Geometry check sheet. Reference: the model listing, model coordinates, mm. Face numbers are marked on the shaded views. A direction names the side the tool comes from. Coordinates: 2 decimals unless noted, no trailing zeros. Write each loop counter-clockwise with the first axis right and the second up, starting at its lowest first coordinate (ties: lowest second). Pieces come first, ordered by that corner, then holes. Notation, with made-up numbers: (35, 34.5) -> (94, 34.5) arc R8 ccw to (94, 38.5) -> close; hole circle Ø7 at (19.25, 16). An arc over 180 degrees is marked (long way). Use a Markdown table: item, result.
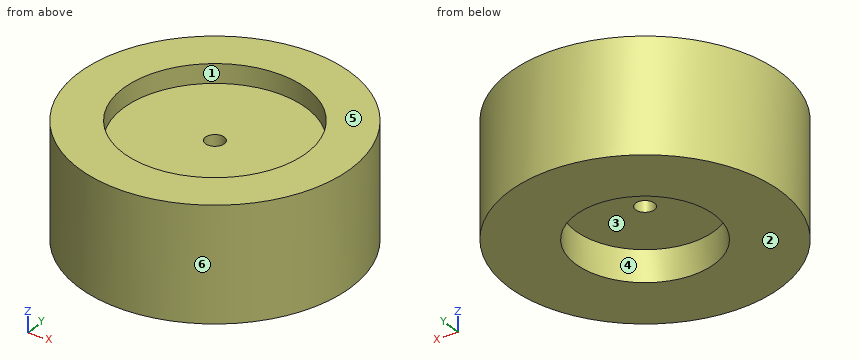
Autodesk Fusion 360 part; units mm, degrees
sketch "Esquisse1" plane through (0, 0, 0) normal (0, 0, 1) x (1, 0, 0)
  circle A0 centre (0, 0) radius 2.15
  dimension "d1" = 4.3
extrude "Extrusion1" add sketch "Esquisse1" along normal blind 1.8
sketch "Esquisse2" plane through (0, 0, 1.8) normal (0, 0, 1) x (-1, 0, 0)
  circle A0 centre (0, 0) radius 2.15
  circle A1 centre (0, 0) radius 1.45
  dimension "d4" = 2.9
extrude "Extrusion2" cut sketch "Esquisse2" against normal blind 0.3 contours A1
sketch "Esquisse3" plane through (0, 0, 0) normal (0, 0, -1) x (1, 0, 0)
  circle A0 centre (0, 0) radius 2.15
  circle A1 centre (0, 0) radius 1.1
  dimension "d7" = 2.2
extrude "Extrusion3" cut sketch "Esquisse3" against normal blind 0.5 contours A1
sketch "Esquisse4" plane through (0, 0, 1.5) normal (0, 0, 1) x (-1, 0, 0)
  circle A0 centre (0, 0) radius 1.45
  circle A1 centre (0, 0) radius 0.15
  dimension "d10" = 0.3
extrude "Extrusion4" cut sketch "Esquisse4" against normal blind 3.8 contours A1
scale "Echelle1" factor 10 about (1.45, 0, 1.8) bodies 1
Item 1: Section check D-D on x = -22. Record the boundary of the cut face in (y, z).
Answer block:
| item | result |
|---|---|
| outline | (-19.55, -16.2) -> (-6.4, -16.2) -> (-6.4, -11.2) -> (6.4, -11.2) -> (6.4, -16.2) -> (19.55, -16.2) -> (19.55, 1.8) -> (11.41, 1.8) -> (11.41, -1.2) -> (-11.41, -1.2) -> (-11.41, 1.8) -> (-19.55, 1.8) -> close |
Item 2: Mould release check, pull along X, two halves, no side actions. Record for the marked faces 4, 5 and 6: +X half, -X half, draft (parallel to the pull), parting line (faces both ways), or undercut.
Answer block:
| item | result |
|---|---|
| face 4 | undercut |
| face 5 | draft |
| face 6 | parting line |
Item 3: Section check A-A on y = 0. Record the boundary of the cut face in (x, z), then the cut area to 3 significant figures.
Answer block:
| item | result |
|---|---|
| outline | (-34.55, -16.2) -> (-24.05, -16.2) -> (-24.05, -11.2) -> (-14.55, -11.2) -> (-14.55, -1.2) -> (-27.55, -1.2) -> (-27.55, 1.8) -> (-34.55, 1.8) -> close; (-11.55, -11.2) -> (-2.05, -11.2) -> (-2.05, -16.2) -> (8.45, -16.2) -> (8.45, 1.8) -> (1.45, 1.8) -> (1.45, -1.2) -> (-11.55, -1.2) -> close |
| area | 547 mm^2 |
Item 4: Thickness scan on L1, parallel to Y at x = -13, z = -5.5; L2, parallel to Y at x = -13.05, z = 0.1; L3, parallel to Z at x = -24.5, y = -6.5. Record the ranges inside material, lowest first. Write a range as [from, to].
Answer block:
| item | result |
|---|---|
| L1 | y = [-21.5, -1.5], [1.5, 21.5] |
| L2 | y = [-21.5, -14.5], [14.5, 21.5] |
| L3 | z = [-16.2, -1.2] |
Item 5: Section check C-C on z = -3.75. Record the boundary of the cut face in (x, y), then the cut area to 3 significant figures.
Answer block:
| item | result |
|---|---|
| outline | circle Ø43 at (-13.05, 0); hole circle Ø3 at (-13.05, 0) |
| area | 1,450 mm^2 |
Item 6: Tool access check on the marked faces 1, 2 and 3. Record the directions out of +Z, -Z, +X, -X, +Y, -Y that give a thin tool (end or side, any length) a straight path to the whole face; none if there is none.
Answer block:
| item | result |
|---|---|
| face 1 | +Z |
| face 2 | -Z, +X, -X, +Y, -Y |
| face 3 | -Z |
Item 7: Depth check by flat-ended pin: P1, Ø2.5, axis at x = -13.05, y = 0, coming from the +Z side; P2, Ø11, axis at x = -8.5, y = -1.5, coming from the -Z side; P3, Ø2, axis at y = 2.5, z = -14, coming from the -X side; P4, Ø2, axis at y = 6, z = -12, coming from the +X side. Enter the tip coordinate at first touch or a pass-through.
Answer block:
| item | result |
|---|---|
| P1 | passes through |
| P2 | stops at z = -11.2 |
| P3 | stops at x = -34.5 |
| P4 | stops at x = 7.86 |
Item 8: Section check B-B on x = -13.05. Record the boundary of the cut face in (y, z).
Answer block:
| item | result |
|---|---|
| outline | (-21.5, -16.2) -> (-11, -16.2) -> (-11, -11.2) -> (-1.5, -11.2) -> (-1.5, -1.2) -> (-14.5, -1.2) -> (-14.5, 1.8) -> (-21.5, 1.8) -> close; (1.5, -11.2) -> (11, -11.2) -> (11, -16.2) -> (21.5, -16.2) -> (21.5, 1.8) -> (14.5, 1.8) -> (14.5, -1.2) -> (1.5, -1.2) -> close |
